Answer from the drawing. Dimensions are ordinates in mm from the lowest x, y and z of the part. A direction names the side the tool comes from. Coordinates: 2 decimals unless noted, no trailing zeros. Order: outer loops, then holes, each group sorted by start corner. A loop starts at its lowest first (then second) coordinate and runs counter-clockwise, first axis right, second up. Notation, with made-up numbers: M 75,85.25 L 83,85.25 A30 ccw 83,121.25 Z; hole C 17,6 d4. An arc over 180 degrees is marked long. Write each question's results on one line, items separated by ' | '.
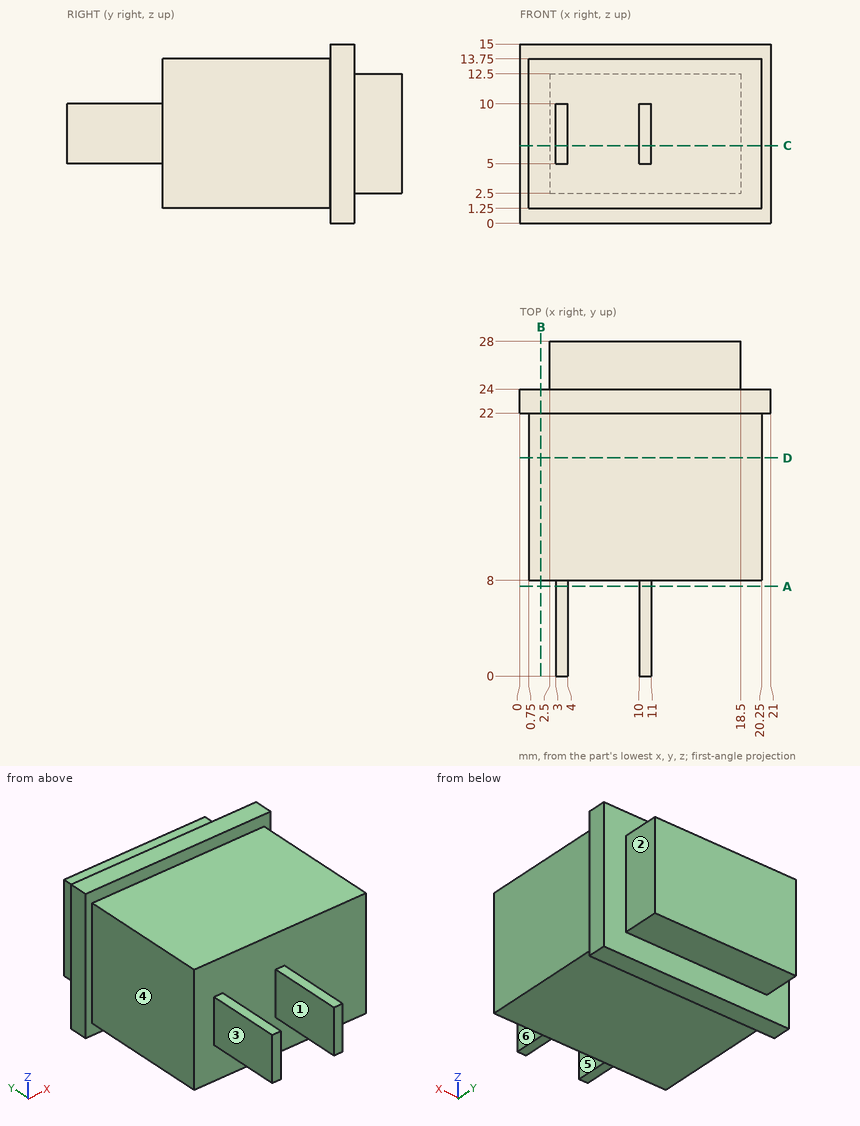
(1) The part is cut by section B-B, the plane x = 1.75. Write down the section's boundary in (y, z), then the cut area to 3 significant figures.
Conclusion:
outline: M 8,1.25 L 22,1.25 L 22,0 L 24,0 L 24,15 L 22,15 L 22,13.75 L 8,13.75 Z | area: 205 mm²
(2) Straight lines are drawn through the part: line 1 (X direction, y = 3.75, z = 5.75); line 2 (Y direction, x = 2.25, z = 11.75); line 3 (X direction, y = 15, z = 9.75). For each, find the intervals that lie inside material, in ascending order.
Conclusion:
line 1: 3 to 4, 10 to 11 | line 2: 8 to 24 | line 3: 0.75 to 20.25
(3) The part is cut by section C-C, the plane z = 6.5. Write down the section's boundary in (x, y).
Conclusion:
outline: M 0,22 L 0.75,22 L 0.75,8 L 3,8 L 3,0 L 4,0 L 4,8 L 10,8 L 10,0 L 11,0 L 11,8 L 20.25,8 L 20.25,22 L 21,22 L 21,24 L 18.5,24 L 18.5,28 L 2.5,28 L 2.5,24 L 0,24 Z
(4) The part is cut by section A-A, the plane y = 7.5. Write down the section's boundary in (x, z), then the cut area to 3 significant figures.
Conclusion:
outline: M 3,5 L 4,5 L 4,10 L 3,10 Z; M 10,5 L 11,5 L 11,10 L 10,10 Z | area: 10.0 mm²
(5) The part is cut by section D-D, the plane y = 18.25. Write down the section's boundary in (x, z), then the cut area to 3 significant figures.
Conclusion:
outline: M 0.75,1.25 L 20.25,1.25 L 20.25,13.75 L 0.75,13.75 Z | area: 244 mm²
(6) Given pin 1 (0.5 mm diameter, centred on x = 10.5, y = 6, fed in from -Z); pin 2 (3 mm diameter, centred on x = 7.5, y = 26, fed in from +Z); pin 3 (2 mm diameter, centred on y = 7.5, z = 3, fed in from +X), each flat-ended and moving along its own axis, determine where each tip first touches the part or whether it passes through.
Conclusion:
pin 1: z = 5 | pin 2: z = 12.5 | pin 3: x = 20.25
(7) The mould has two halves that part along X. Classify the marked faces 1, 2 and 3: pulls with the +X half, pulls with the -X half, needs draft (parallel to the pull), parting line crosses it, or undercut.
Conclusion:
face 1: undercut | face 2: pulls with the +X half | face 3: pulls with the -X half
(8) For the marked faces 4, 5 and 6, determine the directions among +Z, -Z, +X, -X, +Y, -Y from which every point of the face is accessible in a straight line to the end or side of a thin tool.
Conclusion:
face 4: +Z, -Z, -X, -Y | face 5: +Z, -Z, -Y | face 6: +Z, -Z, +X, -Y
